Input: part model. Units: mm. Frame: model coordinates. A direction names the side the tool comes from. Give positions to 0.01 mm unless a question says otherwise; leave off trailing zeros. Loops run counter-clockwise (first coordinate to the right, second up) from the corner with the lowest first, then second, coordinate; pieces in that order, holes last. Notation, with made-up numbers: (-35, -17.5) -> (-2, -17.5) arc R21 ccw to (-2, 18.5) -> close; hole circle Ø9 at (11, 11.25). An arc over 180 degrees is marked (long way). Use CSV: the item, a comma, the result in double quotes.
```python
from build123d import *

# Parameters (mm, degrees)
BOSS_EXTRUDE1_DEPTH            = 4
M3X0_5_TAPPED_HOLE1_D          = 2.5
CBORE_FOR_M3_SHCS1_D           = 3.1
CBORE_FOR_M3_SHCS1_DEPTH       = 4.85
CBORE_FOR_M3_SHCS1_CBORE_D     = 6
CBORE_FOR_M3_SHCS1_CBORE_DEPTH = 3
CBORE_FOR_M3_SHCS1_TIP         = 0.931333959
M3_TAPPED_HOLE1_D              = 2.5
M3_TAPPED_HOLE1_DEPTH          = 5
M3_TAPPED_HOLE1_TIP            = 0.751075774
CHAMFER1_SIZE                  = 2.5
FILLET1_R                      = 2


with BuildPart() as part:
    # Sketch1 → Boss-Extrude1 (new, symmetric)
    with BuildSketch(Plane.XY):
        Polygon((-6.5, 0), (6.5, 0), (6.5, 15.875), (1.65, 15.875), (1.65, 6), (-1.65, 6), (-1.65, 15.875), (-6.5, 15.875), align=None)
    extrude(amount=BOSS_EXTRUDE1_DEPTH, both=True)

    # M3x0.5 Tapped Hole1 (through all)
    with Locations(Plane(origin=(6.5, 0, 0), x_dir=(0, 0, -1), z_dir=(1, 0, 0))):
        with Locations((0, 11.4375)):
            Hole(M3X0_5_TAPPED_HOLE1_D / 2)

    # CBORE for M3 SHCS1
    with Locations(Plane(origin=(6.5, 0, 0), x_dir=(0, 0, -1), z_dir=(1, 0, 0))):
        with Locations((0, 11.4375)):
            CounterBoreHole(CBORE_FOR_M3_SHCS1_D / 2, CBORE_FOR_M3_SHCS1_CBORE_D / 2, CBORE_FOR_M3_SHCS1_CBORE_DEPTH, depth=CBORE_FOR_M3_SHCS1_DEPTH)
            with Locations((0, 0, -(CBORE_FOR_M3_SHCS1_DEPTH + CBORE_FOR_M3_SHCS1_TIP / 2))):  # 118° drill point
                Cone(0, CBORE_FOR_M3_SHCS1_D / 2, CBORE_FOR_M3_SHCS1_TIP, mode=Mode.SUBTRACT)

    # M3 Tapped Hole1
    with Locations(Plane(origin=(0, 0, 0), x_dir=(-1, 0, 0), z_dir=(0, -1, 0))):
        with Locations((0, 0)):
            Hole(M3_TAPPED_HOLE1_D / 2, depth=M3_TAPPED_HOLE1_DEPTH)
            with Locations((0, 0, -(M3_TAPPED_HOLE1_DEPTH + M3_TAPPED_HOLE1_TIP / 2))):  # 118° drill point
                Cone(0, M3_TAPPED_HOLE1_D / 2, M3_TAPPED_HOLE1_TIP, mode=Mode.SUBTRACT)

    # Chamfer1
    chamfer1_edges = [part.edges().sort_by_distance(p)[0] for p in [
        (-1.65, 15.875, 0),
        (1.65, 15.875, 0),
    ]]
    chamfer(chamfer1_edges, length=CHAMFER1_SIZE)

    # Fillet1
    # the kernel refuses this fillet: 2 mm, written as the material it takes off along each edge
    with BuildSketch(Plane(origin=(6.5, -5, -4), x_dir=(-1, 0, 0), z_dir=(0, 1, 0)), Plane(origin=(-6.5, 20.875, 4), x_dir=(0, 0, -1), z_dir=(0, -1, 0)), Plane(origin=(6.5, -5, 4), x_dir=(0, 0, -1), z_dir=(0, 1, 0)), Plane(origin=(-6.5, 20.875, -4), x_dir=(1, 0, 0), z_dir=(0, -1, 0))) as fillet1_piece_1:
        with BuildLine():
            CenterArc((FILLET1_R, FILLET1_R), FILLET1_R, 180, 90)
            Line((0, FILLET1_R), (0, 0))
            Line((0, 0), (FILLET1_R, 0))
        make_face()
    extrude(amount=25.875, mode=Mode.SUBTRACT)


solid = part.part
```
1) Reachability of faces 4 (the cylindrical face through (-0.27, 2.54, 1.22)), 5 (the flat face through (0, 6, 0)), 6 (the flat face through (3.5, 10, -1)) from +Z, -Z, +X, -X, +Y, -Y: full face, straight path, thin tool, end or side. Return the list, or none.
From the geometry:
face 4,"-Y"
face 5,"+Z, -Z, +Y"
face 6,"+X"
2) Section query D-D (x = 5). Return loops of the section in (y, z) (1 decimal), then the cut area to 3 significant figures.
From the geometry:
outline,"(0, -3.9) -> (15.9, -3.9) -> (15.9, 3.9) -> (0, 3.9) -> close; hole circle Ø6 at (11.4, 0)"
area,"96.7 mm^2"
3) Mould query, pull axis Z, two halves, no side actions, for faces 1 (the cylindrical face through (5.021, 11.569, 2.997)), 2 (the flat face through (-5, 15.875, 0)), 3 (the cylindrical face through (-5.93, 8.05, -3.4)). Classes: pulls with the +Z half, pulls with the -Z half, needs draft (parallel to the pull), parting line crosses it, or undercut.
From the geometry:
face 1,"undercut"
face 2,"needs draft"
face 3,"pulls with the -Z half"
4) Contact query for flat-ended pins moving along their axis: pin 1 (1.8 mm diameter, centred on y = 10, z = 1, fed in from +X); pin 2 (1 mm diameter, centred on x = 0, z = -1, fed in from +Y). Output: stop coordinate, or through.
From the geometry:
pin 1,"stops at x = 3.5"
pin 2,"stops at y = 6"
5) Section query A-A (y = 4.75). Return loops of the section in (x, z).
From the geometry:
outline,"(-6.5, -2) arc R2 ccw to (-4.5, -4) -> (4.5, -4) arc R2 ccw to (6.5, -2) -> (6.5, 2) arc R2 ccw to (4.5, 4) -> (-4.5, 4) arc R2 ccw to (-6.5, 2) -> close; hole circle Ø2.5 at (0, 0)"
6) Ray query, line 1 (X direction, y = 7.25, z = -2); line 2 (Y direction, x = 5.25, z = 2) (3 decimals); line 3 (Z direction, x = 0, y = 1.2). Return the intervals inside material, ascending.
From the geometry:
line 1,"x = -6.5 to -1.65, 1.65 to 6.5"
line 2,"y = 0 to 9.201, 13.674 to 15.875"
line 3,"z = -4 to -1.25, 1.25 to 4"
